```python
from build123d import *

# Parameters (mm, degrees)
F1_DEPTH = 65
F2_R     = 1.75
F3_DEPTH = 2.501
F4_R     = 1.75
F5_DEPTH = 2.501


with BuildPart() as f1:
    # F0 (on Right) → F1 (new body)
    with BuildSketch(Plane.YZ):
        Polygon((-17.5, 0), (0, 0), (0, 12.5), (-2.5, 12.5), (-2.5, 2.5), (-17.5, 2.5), align=None)
    extrude(amount=F1_DEPTH)

    # F2 (on face) → F3 (cut, through all)
    with BuildSketch(Plane.XZ.offset(2.5)):
        with Locations((7.5, 9.25)):
            Circle(F2_R)
        with Locations((57.5, 9.25)):
            Circle(F2_R)
    extrude(amount=-F3_DEPTH, mode=Mode.SUBTRACT)

    # F4 (on face) → F5 (cut, through all)
    with BuildSketch(Plane.XY.offset(2.5)):
        with Locations((3.5, -7.25)):
            Circle(F4_R)
        with Locations((61.5, -14.25)):
            Circle(F4_R)
    extrude(amount=-F5_DEPTH, mode=Mode.SUBTRACT)


solid = f1.part
```
Design review of the part built by this model. Coordinates are the model's own, in mm. A direction names the side the tool comes from. Coordinates: 2 decimals unless noted, no trailing zeros. Loops run counter-clockwise (first coordinate to the right, second up) from the corner with the lowest first, then second, coordinate; pieces in that order, holes last.
Q1. We need section B-B on z = 9.25. State the section outline as (x, y) points.
Reported:
outline: (0, -2.5) - (5.75, -2.5) - (5.75, 0) - (0, 0) - close; (9.25, -2.5) - (55.75, -2.5) - (55.75, 0) - (9.25, 0) - close; (59.25, -2.5) - (65, -2.5) - (65, 0) - (59.25, 0) - close
Q2. The part is to be moulded in two halves that separate along Z. For faces 3 (the face through (32, -17.5, 1)), 4 (the face through (32, -10, 2.5)), 5 (the face through (32, -9, 0)), 6 (the face through (8.441, -1.268, 10.726)), say which applies: +Z half, -Z half, draft (parallel to the pull), parting line (faces both ways), or undercut.
Reported:
face 3: draft
face 4: +Z half
face 5: -Z half
face 6: undercut
Q3. We need section A-A on x = 57.5. State the section outline as (y, z) points, and give its area (3 significant figures).
Reported:
outline: (-17.5, 0) - (0, 0) - (0, 7.5) - (-2.5, 7.5) - (-2.5, 2.5) - (-17.5, 2.5) - close; (-2.5, 11) - (0, 11) - (0, 12.5) - (-2.5, 12.5) - close
area: 60.0 mm2
Q4. We need section D-D on z = 1.25. State the section outline as (x, y) points, and give its area (3 significant figures).
Reported:
outline: (0, -17.5) - (65, -17.5) - (65, 0) - (0, 0) - close; hole circle Ø3.5 at (3.5, -7.25); hole circle Ø3.5 at (61.5, -14.25)
area: 1,120 mm2
Q5. To check wall thickness, follow line 1 (Z direction, x = 7.5, y = -0.7); line 2 (Y direction, x = 3.5, z = 1.6); line 3 (Y direction, x = 13, z = 2.75). State the ranges of each line that lie inside material, in increasing order.
Reported:
line 1: z = 0 to 7.5, 11 to 12.5
line 2: y = -17.5 to -9, -5.5 to 0
line 3: y = -2.5 to 0
Q6. For pin 1 (5.5 mm diameter, centred on x = 3.5, y = -7.25, fed in from +Z); pin 2 (2 mm diameter, centred on x = 7.5, z = 9.25, fed in from +Y); pin 3 (6 mm diameter, centred on x = 53, z = 8, fed in from -Y), all flat-tipped, find the tip position at first contact; note any pin that passes through.
Reported:
pin 1: stops at z = 2.5
pin 2: passes through
pin 3: stops at y = -2.5
Q7. Tool access review of faces 1 (the face through (32, -2.5, 8)), 2 (the face through (32, -1, 12.5)): name each direction out of +Z, -Z, +X, -X, +Y, -Y from which nothing blocks a thin tool from reaching the whole face with its end or side.
Reported:
face 1: +Z, +X, -X, -Y
face 2: +Z, +X, -X, +Y, -Y
Q8. We need section C-C on y = -14.25. State the section outline as (x, z) points, and give its area (3 significant figures).
Reported:
outline: (0, 0) - (59.75, 0) - (59.75, 2.5) - (0, 2.5) - close; (63.25, 0) - (65, 0) - (65, 2.5) - (63.25, 2.5) - close
area: 154 mm2
